Autodesk Fusion 360 part; units mm, degrees
sketch "Sketch1" plane through (0, 0, 0) normal (0, 1, 0) x (1, 0, 0)
  line L0 (10, 13) -> (-10, 13) construction
  line L1 (-10, 13) -> (-10, -13) construction
  line L2 (-10, -13) -> (10, -13) construction
  line L3 (10, -13) -> (10, 13) construction
  line L4 (10, 13) -> (-10, -13) construction
  line L5 (-10, 13) -> (10, -13) construction
  circle A0 centre (10, 13) radius 1.5
  line L6 (0, 0) -> (0, 6) construction
  line L7 (0, 0) -> (-6, 0) construction
  line L8 (2.5, 0) -> (20, 0)
  circle A1 centre (10, -13) radius 1.5
  line L9 (0, -20) -> (0, -2.5)
  circle A2 centre (-10, 13) radius 1.5
  circle A3 centre (-10, -13) radius 1.5
  circle A4 centre (-10, -13) radius 3
  circle A5 centre (-10, 13) radius 3
  circle A6 centre (10, -13) radius 3
  circle A7 centre (10, 13) radius 3
  line L10 (15, -18) -> (-15, -18)
  line L11 (-15, -18) -> (-15, 18)
  line L12 (-15, 18) -> (15, 18)
  line L13 (15, 18) -> (15, -18)
  line L14 (15, -18) -> (-15, 18) construction
  line L15 (-15, -18) -> (15, 18) construction
  line L16 (15, -6) -> (27, -6)
  line L17 (27, -6) -> (27, 6)
  line L18 (27, 6) -> (15, 6)
  line L19 (15, 6) -> (15, -6)
  line L20 (15, -6) -> (27, 6) construction
  line L21 (27, -6) -> (15, 6) construction
  circle A8 centre (21, 0) radius 2.75
  circle A9 centre (-21, 0) radius 2.75
  line L22 (-15, -6) -> (-27, -6)
  line L23 (-27, -6) -> (-27, 6)
  line L24 (-27, 6) -> (-15, 6)
  point P0 (21, 0)
  dimension "d1" = 3
  dimension "d2" = 1.5
  dimension "d3" = 26
  dimension "d4" = 20
  dimension "d5" = 5
  dimension "d6" = 5
  dimension "d7" = 12
  dimension "d8" = 12
  dimension "d9" = 5.5
extrude "Extrude1" add sketch "Sketch1" against normal blind 4 contours A0 | L10 L11 L12 L13 L19 | L13 L16 L17 L18 L19 | L11 L22 L23 L24 | A1 | A2 | A3 | A4 | A5 | A6 | A7
extrude "Extrude2" add sketch "Sketch1" along normal blind 5 contours A4 | A5 | A6 | A7
extrude "Extrude3" cut sketch "Sketch1" against normal blind 3 contours A0 | A1 | A2 | A3
fillet "Fillet1" radius 3 8 edges at (-27, -2, -6) (-27, -2, 6) (27, -2, -6) (27, -2, 6) (15, -2, -6) (15, -2, 6) (-15, -2, 6) (-15, -2, -6)
The model under review builds one solid part; all positions refer to its coordinate system, in mm. A direction names the side the tool comes from. Coordinates: 2 decimals unless noted, no trailing zeros. Write each loop counter-clockwise with the first axis right and the second up, starting at its lowest first coordinate (ties: lowest second). Pieces come first, ordered by that corner, then holes. Notation, with made-up numbers: (77.5, 52) - (117.5, 52) arc R19 ccw to (117.5, 67) - close; hole circle Ø2 at (51, 28). An arc over 180 degrees is marked (long way). Write item = value, one per line.
(1) Mouldability with a two-part tool opening along Z and no side actions: class faces 4 (the face through (11.3, 5, 14.3)), 5 (the face through (8.5, 0.94, 13.07)), 6 (the face through (-11.5, 0.94, 13.07)), 7 (the face through (21, -2, 6)) as pulls with the +Z half, pulls with the -Z half, needs draft (parallel to the pull), parting line crosses it, or undercut.
Result sheet:
face_4 = needs draft
face_5 = undercut
face_6 = undercut
face_7 = pulls with the +Z half
(2) Consider section A-A, the plane y = 3. Give the boundary of the cut face in (x, z), then the cut area to 3 significant figures.
Result sheet:
outline = circle Ø6 at (-10, -13); circle Ø6 at (-10, 13); circle Ø6 at (10, -13); circle Ø6 at (10, 13); hole circle Ø3 at (-10, -13); hole circle Ø3 at (-10, 13); hole circle Ø3 at (10, -13); hole circle Ø3 at (10, 13)
area = 84.8 mm^2
(3) Consider section D-D, the plane x = 10. Give the boundary of the cut face in (y, z).
Result sheet:
outline = (-4, -18) - (0, -18) - (0, -16) - (5, -16) - (5, -14.5) - (-3, -14.5) - (-3, -11.5) - (5, -11.5) - (5, -10) - (0, -10) - (0, 10) - (5, 10) - (5, 11.5) - (-3, 11.5) - (-3, 14.5) - (5, 14.5) - (5, 16) - (0, 16) - (0, 18) - (-4, 18) - close
(4) Machinability: for faces 1 (the face through (10, -3, -13)), 2 (the face through (-21, -2, -6)), 3 (the face through (15, -2, -14)), which of the approach directions +Z, -Z, +X, -X, +Y, -Y give a long, thin tool a straight path to every point of the face, cutting with its end or side? Answer none if there is none.
Result sheet:
face_1 = +Y
face_2 = -Z, -X, +Y, -Y
face_3 = -Z, +X, +Y, -Y
(5) For P1, Ø1.8, axis at x = 10, z = 13, coming from the +Y side; P2, Ø1.2, axis at x = -21, y = -3, coming from the -Z side; P3, Ø4.5, axis at x = -22, y = -2, coming from the +Z side, all flat-tipped, find the tip position at first contact; note any pin that passes through.
Result sheet:
P1 = -3
P2 = -6
P3 = 6
(6) For line 1 (Z direction, x = -10, y = 3); line 2 (X direction, y = -1.1, z = 0); line 3 (X direction, y = 3, z = 13), list the stretches that pass through material, from the lowest coordinate up. Write a range as [from, to].
Result sheet:
line_1 = [-16, -14.5], [-11.5, -10], [10, 11.5], [14.5, 16]
line_2 = [-27, -23.75], [-18.25, 18.25], [23.75, 27]
line_3 = [-13, -11.5], [-8.5, -7], [7, 8.5], [11.5, 13]
(7) Consider section B-B, the plane y = -1. Give the boundary of the cut face in (x, z), then the cut area to 3 significant figures.
Result sheet:
outline = (-27, -3) arc R3 ccw to (-24, -6) - (-18, -6) arc R3 cw to (-15, -9) - (-15, -18) - (15, -18) - (15, -9) arc R3 cw to (18, -6) - (24, -6) arc R3 ccw to (27, -3) - (27, 3) arc R3 ccw to (24, 6) - (18, 6) arc R3 cw to (15, 9) - (15, 18) - (-15, 18) - (-15, 9) arc R3 cw to (-18, 6) - (-24, 6) arc R3 ccw to (-27, 3) - close; hole circle Ø5.5 at (-21, 0); hole circle Ø3 at (-10, -13); hole circle Ø3 at (-10, 13); hole circle Ø3 at (10, -13); hole circle Ø3 at (10, 13); hole circle Ø5.5 at (21, 0)
area = 1,290 mm^2
(8) Consider section C-C, the plane z = 13. Give the boundary of the cut face in (x, y), then the cut area to 3 significant figures.
Result sheet:
outline = (-15, -4) - (15, -4) - (15, 0) - (13, 0) - (13, 5) - (11.5, 5) - (11.5, -3) - (8.5, -3) - (8.5, 5) - (7, 5) - (7, 0) - (-7, 0) - (-7, 5) - (-8.5, 5) - (-8.5, -3) - (-11.5, -3) - (-11.5, 5) - (-13, 5) - (-13, 0) - (-15, 0) - close
area = 132 mm^2
